The model under review builds one solid part; all positions refer to its coordinate system, in mm. Face numbers are marked on the shaded views. A direction names the side the tool comes from. Coordinates: 2 decimals unless noted, no trailing zeros. Order: outer loops, then holes, each group sorted by start corner. A loop starts at its lowest first (then second) coordinate and runs counter-clockwise, first axis right, second up. Notation, with made-up numbers: (-5, -30) -> (2, -30) arc R5 cw to (2, -26) -> close; hole circle Ø8 at (69, 88). An arc over 180 degrees is marked (long way). Put each result on its own line as item: value.
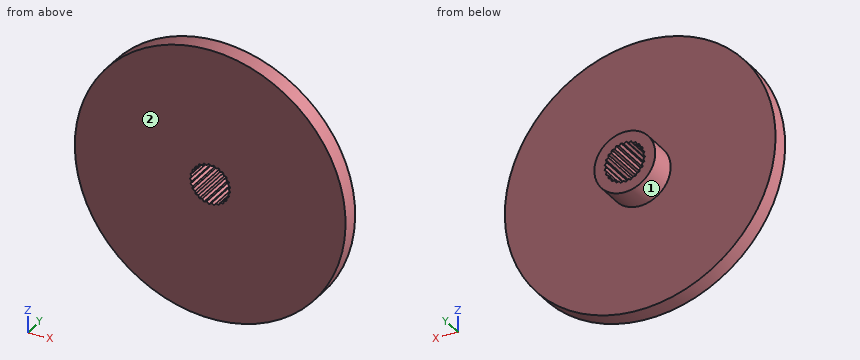
from build123d import *

# Parameters (mm, degrees)
SKETCH2_R               = 20
BOSS_EXTRUDE1_DEPTH     = 2.5
SKETCH3_R               = 4.5
SKETCH3_R_2             = 2.75
BOSS_EXTRUDE2_DEPTH     = 4
CUT_EXTRUDE1_DEPTH      = 29.565713714
CUT_EXTRUDE1_DEPTH_BACK = 29.565713714
SKETCH3_3_R             = 2.75
CUT_EXTRUDE2_DEPTH      = 30.021543722
CIRPATTERN1_COUNT       = 25


with BuildPart() as part:
    # Sketch2 → Boss-Extrude1 (new body)
    with BuildSketch(Plane(origin=(0, 0, 0), x_dir=(1, 0, 0), z_dir=(0, 1, 0))):
        with Locations(Location((0, 0, 0), (0, 0, 270))):
            Circle(SKETCH2_R)
    extrude(amount=BOSS_EXTRUDE1_DEPTH)

    # Sketch3 → Boss-Extrude2 (add)
    with BuildSketch(Plane(origin=(0, 2.5, 0), x_dir=(1, 0, 0), z_dir=(0, 1, 0))):
        with Locations(Location((0, 0, 0), (0, 0, 270))):
            Circle(SKETCH3_R)
        with Locations(Location((0, 0, 0), (0, 0, 270))):
            Circle(SKETCH3_R_2, mode=Mode.SUBTRACT)
    extrude(amount=BOSS_EXTRUDE2_DEPTH)

    # Sketch3_3 → Cut-Extrude1 (cut, two sides: drawn at the far end of the back side and taken through both)
    with BuildSketch(Plane(origin=(0, 2.5, 0), x_dir=(1, 0, 0), z_dir=(0, 1, 0)).offset(-CUT_EXTRUDE1_DEPTH_BACK)):
        with Locations(Location((0, 0, 0), (0, 0, 270))):
            Circle(SKETCH3_3_R)
    extrude(amount=CUT_EXTRUDE1_DEPTH + CUT_EXTRUDE1_DEPTH_BACK, mode=Mode.SUBTRACT)

    # Sketch5 → Cut-Extrude2 (cut, symmetric)
    with BuildSketch(Plane(origin=(0, 6.5, 0), x_dir=(1, 0, 0), z_dir=(0, 1, 0))):
        with BuildLine():
            ThreePointArc((0.160191529, -2.74533034), (-0.185152758, -2.743759912), (-0.527577075, -2.698918752))
            Line((-0.527577075, -2.698918752), (-0.201984827, -2.993192632))
            Line((-0.201984827, -2.993192632), (0.160191529, -2.74533034))
        make_face()
    cut_extrude2 = extrude(amount=CUT_EXTRUDE2_DEPTH, both=True, mode=Mode.SUBTRACT)

    # CirPattern1: Cut-Extrude2 ×25 about axis
    cirpattern1_axis = Axis((0, 0, 0), (0, 1, 0))
    for i in range(1, CIRPATTERN1_COUNT):
        add(cut_extrude2.rotate(cirpattern1_axis, i * 360 / CIRPATTERN1_COUNT), mode=Mode.SUBTRACT)


solid = part.part
Item 1: For pin 1 Ø1.5 at (y, z) = (1.5, 9.5) entering from -X; pin 2 Ø1 at (x, z) = (12, 4.5) entering from +Y; pin 3 Ø3 at (y, z) = (3.5, -3.5) entering from +X, all flat-tipped, find the tip position at first contact; note any pin that passes through.
Answers below:
pin 1: x = -17.98
pin 2: y = 2.5
pin 3: x = 19.86
Item 2: Consider section A-A on z = 17. Write out the cut boundary in (x, y).
Answers below:
outline: (-10.54, 0) -> (10.54, 0) -> (10.54, 2.5) -> (-10.54, 2.5) -> close
Item 3: Consider section B-B on x = 11. Write out the cut boundary in (y, z).
Answers below:
outline: (0, -16.7) -> (2.5, -16.7) -> (2.5, 16.7) -> (0, 16.7) -> close
Item 4: For the marked faces 1 and 2, list the 3-axis set-ups (+Z, -Z, +X, -X, +Y, -Y) from which the entire face can be reached by the end or side of a thin tool; tool diameter is ignored.
Answers below:
face 1: +Y
face 2: +Z, -Z, +X, -X, -Y
Item 5: For line 1 (Y direction, x = 10.5, z = 7.5); line 2 (Z direction, x = -1.5, y = 5.5); line 3 (Z direction, x = -8, y = 1.5), list the stretches that pass through material, from the lowest coordinate up. Write a range as from..to.
Answers below:
line 1: 0..2.5
line 2: -4.24..-2.53, 2.51..4.24
line 3: -18.33..18.33
